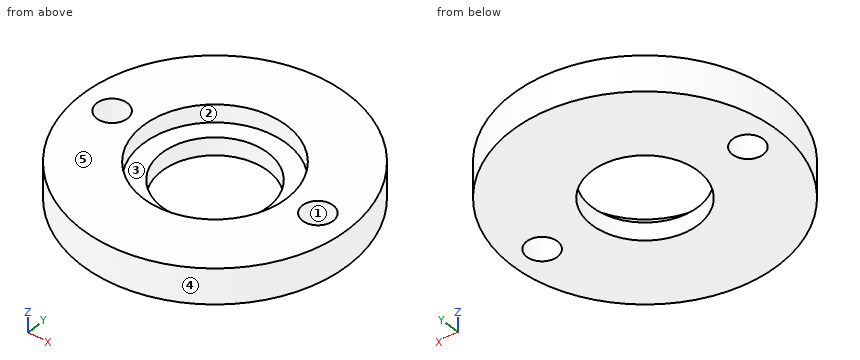
from build123d import *

# Parameters (mm, degrees)
SKETCH1_R           = 15
SKETCH1_R_2         = 6
SKETCH1_R_3         = 1.725
BOSS_EXTRUDE1_DEPTH = 4
CUT_EXTRUDE1_START  = -2
SKETCH2_R           = 8.1
SKETCH2_R_2         = 6
CUT_EXTRUDE1_DEPTH  = 2


with BuildPart() as part:
    # Sketch1 → Boss-Extrude1 (new body)
    with BuildSketch(Plane.XY):
        Circle(SKETCH1_R)
        Circle(SKETCH1_R_2, mode=Mode.SUBTRACT)
        with Locations((-11.5, 0)):
            Circle(SKETCH1_R_3, mode=Mode.SUBTRACT)
        with Locations((11.5, 0)):
            Circle(SKETCH1_R_3, mode=Mode.SUBTRACT)
    extrude(amount=BOSS_EXTRUDE1_DEPTH)

    # Sketch2 → Cut-Extrude1 (cut)
    with BuildSketch(Plane.XY.offset(4).offset(CUT_EXTRUDE1_START)):
        Circle(SKETCH2_R)
        Circle(SKETCH2_R_2, mode=Mode.SUBTRACT)
    extrude(amount=CUT_EXTRUDE1_DEPTH, mode=Mode.SUBTRACT)


solid = part.part
Part model, mm, in its own coordinate system. Face numbers are marked on the shaded views. A direction names the side the tool comes from. Coordinates: 2 decimals unless noted, no trailing zeros. Order: outer loops, then holes, each group sorted by start corner. A loop starts at its lowest first (then second) coordinate and runs counter-clockwise, first axis right, second up. Notation, with made-up numbers: M 33.5,32.5 L 48.5,32.5 A10 cw 48.5,36.5 Z; hole C 26.5,-24 d8. An arc over 180 degrees is marked long. Use a Markdown table: item, result.
(1) Pull direction Y, two halves, no side cores. Call the marked faces 3, 4 and 5: released by +Y, released by -Y, zero draft, split by the parting line, or undercut.
A:
| item | result |
|---|---|
| face 3 | undercut |
| face 4 | split by the parting line |
| face 5 | zero draft |
(2) Flat gauge pins, fed straight in: pin 1 (2 mm diameter, centred on x = -4.5, z = 1, fed in from +Y); pin 2 (3 mm diameter, centred on x = 11.5, y = 0, fed in from -Z); pin 3 (1.5 mm diameter, centred on x = -10, z = 1.5, fed in from +Y). Where does each tip first touch, or does it go through?
A:
| item | result |
|---|---|
| pin 1 | stops at y = 14.59 |
| pin 2 | passes through |
| pin 3 | stops at y = 11.81 |
(3) Cut at C-C on y = -4.5. Write the cut outline in (x, z), then the cut area to 3 significant figures.
A:
| item | result |
|---|---|
| outline | M -14.31,0 L -3.97,0 L -3.97,2 L -6.73,2 L -6.73,4 L -14.31,4 Z; M 3.97,0 L 14.31,0 L 14.31,4 L 6.73,4 L 6.73,2 L 3.97,2 Z |
| area | 71.7 mm^2 |
(4) Cut at B-B on y = 0. Write the cut outline in (x, z) (3 decimals).
A:
| item | result |
|---|---|
| outline | M -15,0 L -13.225,0 L -13.225,4 L -15,4 Z; M -9.775,0 L -6,0 L -6,2 L -8.1,2 L -8.1,4 L -9.775,4 Z; M 6,0 L 9.775,0 L 9.775,4 L 8.1,4 L 8.1,2 L 6,2 Z; M 13.225,0 L 15,0 L 15,4 L 13.225,4 Z |
(5) Cut at A-A on x = 0. Write the cut outline in (y, z), then the cut area to 3 significant figures.
A:
| item | result |
|---|---|
| outline | M -15,0 L -6,0 L -6,2 L -8.1,2 L -8.1,4 L -15,4 Z; M 6,0 L 15,0 L 15,4 L 8.1,4 L 8.1,2 L 6,2 Z |
| area | 63.6 mm^2 |
(6) Cut at D-D on z = 3. Write the cut outline in (x, y) (3 decimals).
A:
| item | result |
|---|---|
| outline | C 0,0 d30; hole C -11.5,0 d3.45; hole C 0,0 d16.2; hole C 11.5,0 d3.45 |
(7) Probe L1, parallel to Y at x = 0, z = 1.65; L2, parallel to X at y = 1, z = 0.25; L3, parallel to Y at x = -11.5, z = 2.3 (3 decimals). List the from-to ranges inside material, lowest first.
A:
| item | result |
|---|---|
| L1 | y = -15 to -6, 6 to 15 |
| L2 | x = -14.97 to -12.91, -10.09 to -5.92, 5.92 to 10.09, 12.91 to 14.97 |
| L3 | y = -9.631 to -1.725, 1.725 to 9.631 |
(8) Tool access for the marked faces 1 and 2: list every direction of +Z, -Z, +X, -X, +Y, -Y with a clear straight run to the whole face (end or side of a thin tool).
A:
| item | result |
|---|---|
| face 1 | +Z, -Z |
| face 2 | +Z |
